```python
from build123d import *

# Parameters (mm, degrees)
F1_DEPTH = 2
F2_R     = 2
F3_DEPTH = 5


with BuildPart() as f1:
    # F0 (on Top) → F1 (new body)
    with BuildSketch(Plane.XY):
        with BuildLine():
            Line((0.68328, -6.032679), (-7.31672, -6.032679))
            ThreePointArc((-7.31672, -6.032679), (-8.023827, -6.325572), (-8.31672, -7.032679))
            Line((-8.31672, -7.032679), (-8.31672, -10.032679))
            ThreePointArc((-8.31672, -10.032679), (-8.023827, -10.739785), (-7.31672, -11.032679))
            Line((-7.31672, -11.032679), (0.68328, -11.032679))
            ThreePointArc((0.68328, -11.032679), (1.390386, -10.739785), (1.68328, -10.032679))
            Line((1.68328, -10.032679), (1.68328, -7.032679))
            ThreePointArc((1.68328, -7.032679), (1.390386, -6.325572), (0.68328, -6.032679))
        make_face()
    extrude(amount=F1_DEPTH)

    # F2 (on face) → F3 (join)
    with BuildSketch(Plane.XY.offset(2)):
        with Locations((-3.31672, -8.532679)):
            Circle(F2_R)
    extrude(amount=F3_DEPTH)


solid = f1.part
```
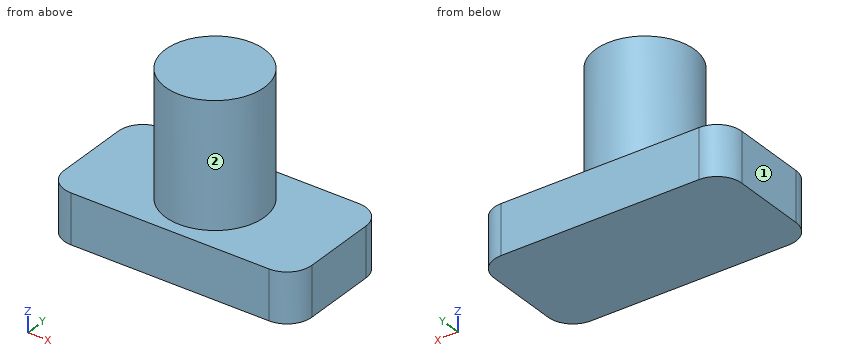
CAD build for the part. Positions are in the model's coordinates, mm. Face numbers are marked on the shaded views. A direction names the side the tool comes from. Coordinates: 2 decimals unless noted, no trailing zeros. Write each loop counter-clockwise with the first axis right and the second up, starting at its lowest first coordinate (ties: lowest second). Pieces come first, ordered by that corner, then holes. Notation, with made-up numbers: (-1.5, 63) -> (52.5, 63) arc R8 cw to (52.5, 71) -> close; hole circle Ø9 at (2.25, 66). An arc over 180 degrees is marked (long way). Use CSV: the item, a comma, the result in double quotes. Start each with the question number.
Item 1: Drop flat-ended pins along their axis: P1, Ø3, axis at x = -5.5, z = 4, coming from the -Y side; P2, Ø1.5, axis at x = -1.5, z = 5.5, coming from the +Y side. Give the stop position or say it passes through.
Item 2: Band-saw the part on D-D, the plane z = 2.25. Write the cut outline in (x, y).
Item 3: Band-saw the part on B-B, the plane y = -9.35. Write the cut outline in (x, z), plus the area to 3 significant figures.
Item 4: Band-saw the part on C-C, the plane x = 0.25. Write the cut outline in (y, z).
Item 5: Wall check: probe 1 along X at (y, z) = (-8.65, 4.25); probe 2 along Z at (x, y) = (-7, -8.75); probe 3 along X at (y, z) = (-8.1, 3.5). Give the ranges that are in metal, low to high.
Item 6: Tool access for the marked faces 1 and 2: list every direction of +Z, -Z, +X, -X, +Y, -Y with a clear straight run to the whole face (end or side of a thin tool).
Item 7: Band-saw the part on A-A, the plane z = 0.5. Write the cut outline in (x, y), plus the area to 3 significant figures.
Response values:
1,P1,"stops at y = -10.41"
1,P2,"stops at y = -6.84"
2,outline,"circle Ø4 at (-3.32, -8.53)"
3,outline,"(-8.32, 0) -> (1.68, 0) -> (1.68, 2) -> (-1.49, 2) -> (-1.49, 7) -> (-5.14, 7) -> (-5.14, 2) -> (-8.32, 2) -> close"
3,area,"38.3 mm2"
4,outline,"(-11.03, 0) -> (-6.03, 0) -> (-6.03, 2) -> (-11.03, 2) -> close"
5,probe 1,"x = -5.31 to -1.32"
5,probe 2,"z = 0 to 2"
5,probe 3,"x = -5.27 to -1.36"
6,face 1,"+Z, -Z, -X, +Y, -Y"
6,face 2,"+Z"
7,outline,"(-8.32, -10.03) arc R1 ccw to (-7.32, -11.03) -> (0.68, -11.03) arc R1 ccw to (1.68, -10.03) -> (1.68, -7.03) arc R1 ccw to (0.68, -6.03) -> (-7.32, -6.03) arc R1 ccw to (-8.32, -7.03) -> close"
7,area,"49.1 mm2"
